Check sheet for the modelled part. Datum: model origin and axes. Units: mm. Face numbers are marked on the shaded views. Give positions to 0.01 mm unless a question says otherwise; leave off trailing zeros. Order: outer loops, then holes, each group sorted by start corner. A loop starts at its lowest first (then second) coordinate and runs counter-clockwise, first axis right, second up.
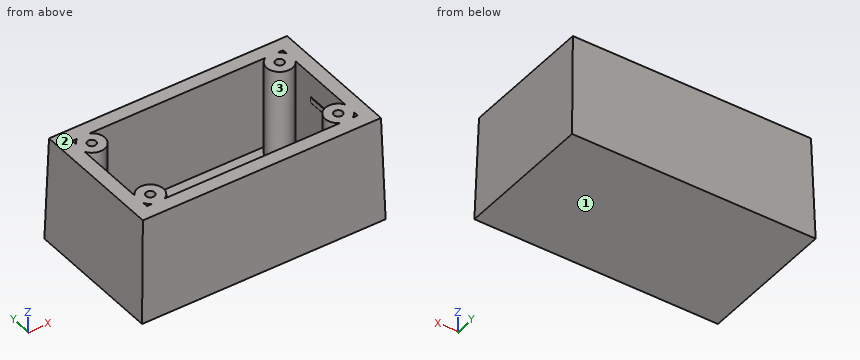
```python
from build123d import *

# Parameters (mm, degrees)
SKETCH2_W                 = 70
SKETCH2_H                 = 40
DRAFTED_OUTER_SHELL_DEPTH = 30
DRAFTED_OUTER_SHELL_TAPER = 1.5
DRAFTED_CAVITY_START      = 3
SKETCH3_W                 = 62
SKETCH3_H                 = 32
DRAFTED_CAVITY_DEPTH      = 27
DRAFTED_CAVITY_TAPER      = 1.5
SCREW_BOSS_START          = 3
SKETCH4_R                 = 3.75
SCREW_BOSS_DEPTH          = 27
SCREW_BOSS_BORE_START     = 3
SKETCH5_R                 = 1.25
SCREW_BOSS_BORE_DEPTH     = 27
BOSS_EXTRUDE3_START       = 3
SKETCH6_R                 = 3.75
BOSS_EXTRUDE3_DEPTH       = 27
CUT_EXTRUDE3_START        = 3
SKETCH7_R                 = 1.25
CUT_EXTRUDE3_DEPTH        = 27
BOSS_EXTRUDE4_START       = 3
SKETCH8_R                 = 3.75
BOSS_EXTRUDE4_DEPTH       = 27
CUT_EXTRUDE4_START        = 3
SKETCH9_R                 = 1.25
CUT_EXTRUDE4_DEPTH        = 27
BOSS_EXTRUDE5_START       = 3
SKETCH10_R                = 3.75
BOSS_EXTRUDE5_DEPTH       = 27
CUT_EXTRUDE5_START        = 3
SKETCH11_R                = 1.25
CUT_EXTRUDE5_DEPTH        = 27
SNAP_CATCH_LEDGE_START    = 21.6
SKETCH12_W                = 2.107019882
SKETCH12_H                = 8
SNAP_CATCH_LEDGE_DEPTH    = 1.5
BOSS_EXTRUDE7_START       = 21.6
SKETCH13_W                = 2.107019882
SKETCH13_H                = 8
BOSS_EXTRUDE7_DEPTH       = 1.5


with BuildPart() as part:
    # Sketch2 → Drafted_outer_shell (new body)
    with BuildSketch(Plane.XY):
        Rectangle(SKETCH2_W, SKETCH2_H)
    extrude(amount=DRAFTED_OUTER_SHELL_DEPTH, taper=DRAFTED_OUTER_SHELL_TAPER)

    # Sketch3 → Drafted_cavity (cut)
    with BuildSketch(Plane.XY.offset(DRAFTED_CAVITY_START)):
        Rectangle(SKETCH3_W, SKETCH3_H)
    extrude(amount=DRAFTED_CAVITY_DEPTH, taper=DRAFTED_CAVITY_TAPER, mode=Mode.SUBTRACT)

    # Sketch4 → Screw_boss (add)
    with BuildSketch(Plane.XY.offset(SCREW_BOSS_START)):
        with Locations(Location((-27, -12, 0), (0, 0, 180))):
            Circle(SKETCH4_R)
    extrude(amount=SCREW_BOSS_DEPTH)

    # Sketch5 → Screw_boss_bore (cut)
    with BuildSketch(Plane.XY.offset(SCREW_BOSS_BORE_START)):
        with Locations((-27, -12)):
            Circle(SKETCH5_R)
    extrude(amount=SCREW_BOSS_BORE_DEPTH, mode=Mode.SUBTRACT)

    # Sketch6 → Boss-Extrude3 (add)
    with BuildSketch(Plane.XY.offset(BOSS_EXTRUDE3_START)):
        with Locations(Location((-27, 12, 0), (0, 0, 180))):
            Circle(SKETCH6_R)
    extrude(amount=BOSS_EXTRUDE3_DEPTH)

    # Sketch7 → Cut-Extrude3 (cut)
    with BuildSketch(Plane.XY.offset(CUT_EXTRUDE3_START)):
        with Locations((-27, 12)):
            Circle(SKETCH7_R)
    extrude(amount=CUT_EXTRUDE3_DEPTH, mode=Mode.SUBTRACT)

    # Sketch8 → Boss-Extrude4 (add)
    with BuildSketch(Plane.XY.offset(BOSS_EXTRUDE4_START)):
        with Locations(Location((27, -12, 0), (0, 0, 180))):
            Circle(SKETCH8_R)
    extrude(amount=BOSS_EXTRUDE4_DEPTH)

    # Sketch9 → Cut-Extrude4 (cut)
    with BuildSketch(Plane.XY.offset(CUT_EXTRUDE4_START)):
        with Locations((27, -12)):
            Circle(SKETCH9_R)
    extrude(amount=CUT_EXTRUDE4_DEPTH, mode=Mode.SUBTRACT)

    # Sketch10 → Boss-Extrude5 (add)
    with BuildSketch(Plane.XY.offset(BOSS_EXTRUDE5_START)):
        with Locations(Location((27, 12, 0), (0, 0, 180))):
            Circle(SKETCH10_R)
    extrude(amount=BOSS_EXTRUDE5_DEPTH)

    # Sketch11 → Cut-Extrude5 (cut)
    with BuildSketch(Plane.XY.offset(CUT_EXTRUDE5_START)):
        with Locations((27, 12)):
            Circle(SKETCH11_R)
    extrude(amount=CUT_EXTRUDE5_DEPTH, mode=Mode.SUBTRACT)

    # Sketch12 → Snap_catch_ledge (add)
    with BuildSketch(Plane.XY.offset(SNAP_CATCH_LEDGE_START)):
        with Locations((-31.346490059, 0)):
            Rectangle(SKETCH12_W, SKETCH12_H)
    extrude(amount=SNAP_CATCH_LEDGE_DEPTH)

    # Sketch13 → Boss-Extrude7 (add)
    with BuildSketch(Plane.XY.offset(BOSS_EXTRUDE7_START)):
        with Locations((31.346490059, 0)):
            Rectangle(SKETCH13_W, SKETCH13_H)
    extrude(amount=BOSS_EXTRUDE7_DEPTH)


solid = part.part
```
(1) Sectioned sample at B-B (y = -7.5). Enter the section's corners in (x, z).
(2) Go/stop test with flat-tipped pins: P1, Ø1.5, axis at x = -2, z = 10.5, coming from the +Y side; P2, Ø6, axis at x = 24.5, z = 23.5, coming from the -Y side; P3, Ø9.5, axis at x = 10.5, y = 5, coming from the +Z side. Record where each tip stops, or that it passes through.
(3) Sectioned sample at A-A (z = 4). Count the separate pieces of the cut face and the enclosed holes in it, plus the area to 3 significant figures.
(4) Release check for a two-part mould opening along Z. For the marked faces 1, 2 and 3 record: released by +Z, released by -Z, zero draft, split by the parting line, or undercut.
(5) Sectioned sample at C-C (x = 27). Enter the section's corners in (y, z), plus the area to 3 significant figures.
(6) Thickness scan on L1, parallel to X at y = 14.5, z = 22; L2, parallel to Y at x = 27, z = 22.5; L3, parallel to Y at x = 27, z = 17. Record the ranges inside material, lowest first.
Values follow:
1. outline: (-35, 0) - (35, 0) - (34.21, 30) - (30.29, 30) - (31, 3) - (-31, 3) - (-30.29, 30) - (-34.21, 30) - close
2. P1: stops at y = 19.74
2. P2: stops at y = -19.46
2. P3: stops at z = 3
3. separate pieces: 5
3. enclosed holes: 5
3. area: 955 mm2
4. face 1: released by -Z
4. face 2: released by +Z
4. face 3: undercut
5. outline: (-20, 0) - (20, 0) - (19.21, 30) - (13.25, 30) - (13.25, 3) - (10.75, 3) - (10.75, 30) - (8.25, 30) - (8.25, 3) - (-8.25, 3) - (-8.25, 30) - (-10.75, 30) - (-10.75, 3) - (-13.25, 3) - (-13.25, 30) - (-19.21, 30) - close; hole (-16, 3) - (-15.75, 3) - (-15.75, 12.55) - close; hole (15.75, 3) - (16, 3) - (15.75, 12.55) - close
5. area: 594 mm2
6. L1: x = -34.42 to -30.5, -29.8 to -24.2, 24.2 to 29.8, 30.5 to 34.42
6. L2: y = -19.41 to -13.25, -10.75 to -8.25, 8.25 to 10.75, 13.25 to 19.41
6. L3: y = -19.55 to -13.25, -10.75 to -8.25, 8.25 to 10.75, 13.25 to 19.55
